from build123d import *

# Parameters (mm, degrees)
F0_W     = 378.75718
F0_H     = 914.4
F1_DEPTH = 25.4
F3_DEPTH = 25.401
F4_R     = 33.437192
F5_DEPTH = 25.4


with BuildPart() as f1:
    # F0 (on Top) → F1 (new body)
    with BuildSketch(Plane.XY):
        with Locations((-4.136321, 70.025934)):
            Rectangle(F0_W, F0_H)
    extrude(amount=F1_DEPTH)

    # F2 (on face) → F3 (cut, through all)
    with BuildSketch(Plane.XY.offset(25.4)):
        with BuildLine():
            Line((-142.714911, 514.525934), (-142.714911, 511.350934))
            ThreePointArc((-142.714911, 511.350934), (-140.469847, 512.28087), (-139.539911, 514.525934))
            ThreePointArc((-139.539911, 514.525934), (-140.469847, 516.770998), (-142.714911, 517.700934))
            Line((-142.714911, 517.700934), (-142.714911, 514.525934))
        make_face()
        with BuildLine():
            ThreePointArc((-142.714911, 517.700934), (-145.889911, 514.525934), (-142.714911, 511.350934))
            Line((-142.714911, 511.350934), (-142.714911, 514.525934))
            Line((-142.714911, 514.525934), (-142.714911, 517.700934))
        make_face()
        with BuildLine():
            Line((134.442269, 514.525934), (134.442269, 511.350934))
            ThreePointArc((134.442269, 511.350934), (136.687333, 512.28087), (137.617269, 514.525934))
            ThreePointArc((137.617269, 514.525934), (136.687333, 516.770998), (134.442269, 517.700934))
            Line((134.442269, 517.700934), (134.442269, 514.525934))
        make_face()
        with BuildLine():
            ThreePointArc((134.442269, 517.700934), (131.267269, 514.525934), (134.442269, 511.350934))
            Line((134.442269, 511.350934), (134.442269, 514.525934))
            Line((134.442269, 514.525934), (134.442269, 517.700934))
        make_face()
        with BuildLine():
            ThreePointArc((-142.714911, -377.649066), (-140.469847, -376.71913), (-139.539911, -374.474066))
            ThreePointArc((-139.539911, -374.474066), (-144.959975, -372.229002), (-142.714911, -377.649066))
        make_face()
        with BuildLine():
            ThreePointArc((134.442269, -377.649066), (136.687333, -376.71913), (137.617269, -374.474066))
            ThreePointArc((137.617269, -374.474066), (136.687333, -372.229002), (134.442269, -371.299066))
            Line((134.442269, -371.299066), (134.442269, -374.474066))
            Line((134.442269, -374.474066), (134.442269, -377.649066))
        make_face()
        with BuildLine():
            Line((134.442269, -374.474066), (134.442269, -371.299066))
            ThreePointArc((134.442269, -371.299066), (131.267269, -374.474066), (134.442269, -377.649066))
            Line((134.442269, -377.649066), (134.442269, -374.474066))
        make_face()
    extrude(amount=-F3_DEPTH, mode=Mode.SUBTRACT)

    # F4 (on face) → F5 (cut)
    with BuildSketch(Plane.XY.offset(25.4)):
        with Locations((-2.0491, 74.617796)):
            Circle(F4_R)
    extrude(amount=-F5_DEPTH, mode=Mode.SUBTRACT)


solid = f1.part
The listing builds one solid part. Answer for the finished solid, in the listing's coordinates (mm). Give positions to 0.01 mm unless a question says otherwise; leave off trailing zeros. Write each loop counter-clockwise with the first axis right and the second up, starting at its lowest first coordinate (ties: lowest second). Pieces come first, ordered by that corner, then holes.
Item 1: Section A-A, the plane x = -13 is taken. Write down the section's boundary in (y, z).
Item 2: Find the intervals of material crossed by line 1 along X through (y, z) = (63, 12.25); line 2 along Y through (x, z) = (19.5, 12.25) (3 decimals); line 3 along Y through (x, z) = (17, 17.75), in increasing order.
Item 3: A flat-ended cylindrical pin translates along its axis: P1, Ø1, axis at x = -64, y = 211.5, coming from the -Z side. Find the tip coordinate at first contact, or state that the pin passes through.
Item 4: Section B-B, the plane y = 59.5 is taken. Write down the section's boundary in (x, z), plus the area to 3 significant figures.
Item 5: Determine the mould class of faces 1 (the cylindrical face through (-6.4, 107.77, 12.88)), 2 (the flat face through (-7, 527.226, 13)), 3 (the flat face through (-49, 76, 0)), 4 (the flat face through (-7, -387.174, 13)) for opening direction Y: released by +Y, released by -Y, zero draft, split by the parting line, or undercut.
Completed:
1. outline: (-387.17, 0) - (43.02, 0) - (43.02, 25.4) - (-387.17, 25.4) - close; (106.21, 0) - (527.23, 0) - (527.23, 25.4) - (106.21, 25.4) - close
2. line 1: x = -193.51 to -33.4, 29.3 to 185.24
2. line 2: y = -387.174 to 49.051, 100.185 to 527.226
2. line 3: y = -387.17 to 47.14, 102.1 to 527.23
3. P1: stops at z = 0
4. outline: (-193.51, 0) - (-31.87, 0) - (-31.87, 25.4) - (-193.51, 25.4) - close; (27.78, 0) - (185.24, 0) - (185.24, 25.4) - (27.78, 25.4) - close
4. area: 8,110 mm2
5. face 1: undercut
5. face 2: released by +Y
5. face 3: zero draft
5. face 4: released by -Y
